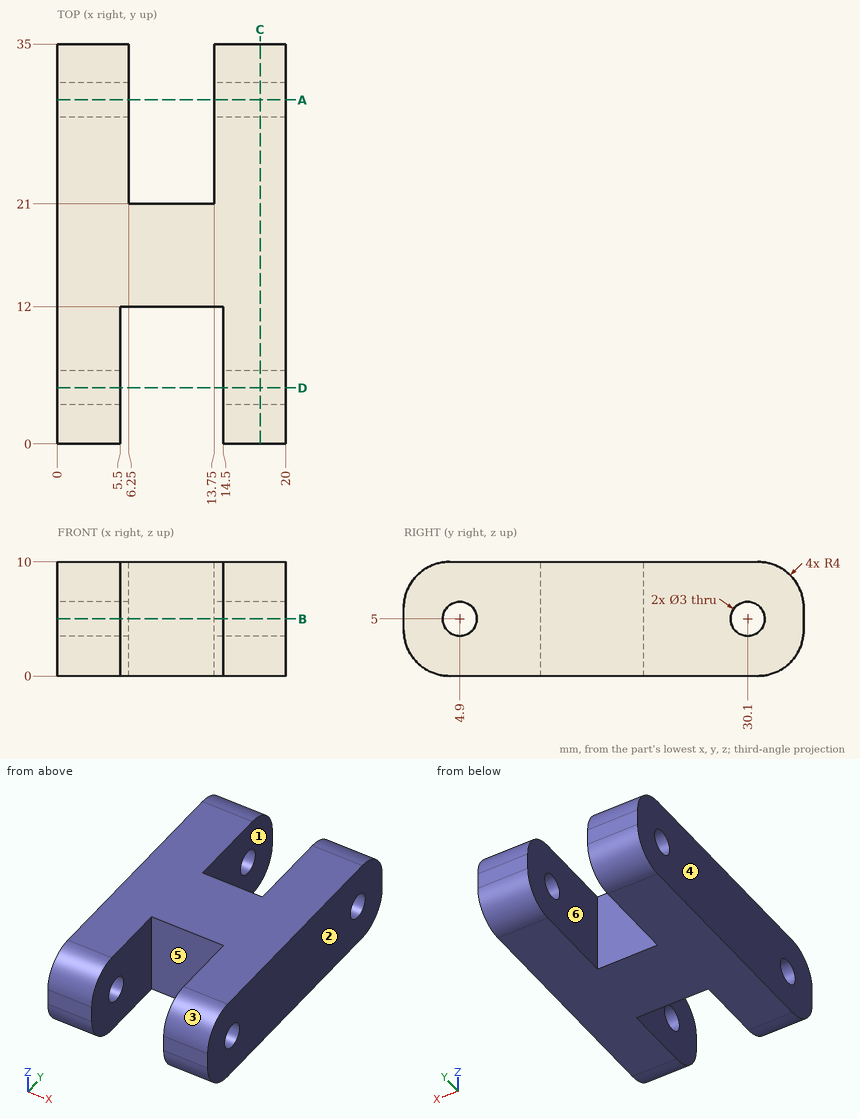
Could you check a few things on this drawing? It's one solid part, dimensions in mm from its lowest x, y, z. A direction names the side the tool comes from. Give positions to 0.01 mm unless a question says otherwise; leave off trailing zeros. Loops run counter-clockwise (first coordinate to the right, second up) from the corner with the lowest first, then second, coordinate; pieces in that order, holes last. Notation, with made-up numbers: M -38.75,12.25 L 1.25,12.25 A14 cw 1.25,19.25 Z; hole C 22.25,8.25 d5. An arc over 180 degrees is marked long. One line per question, with ' | ' between items. Start each with the question number.
Q1. If I drill on line 1 (Y direction, x = 4.15, z = 5); line 2 (Z direction, x = 3.5, y = 30.1); line 3 (X direction, y = 4.5, z = 9.75), over which ranges is the centre line in solid material (lowest first)? Write a range as from..to.
Q2. For the marked faces 4, 5 and 6, which set-ups out of +Z, -Z, +X, -X, +Y, -Y let a thin tool reach every point of the face, with its end or its side?
Q3. If we section it at C-C (x = 17.75): Please give me the cut outline in (y, z).
Q4. If we section it at B-B (z = 5): Please give me the cut outline in (x, y).
Q5. If we section it at A-A (y = 30.1): Please give me the cut outline in (x, z), plus the area to 3 significant figures.
Q6. If we mould it in two halves opening along X, with no side actions, what happens to the marked faces 1, 2 and 3? For each: +X half, -X half, draft (parallel to the pull), parting line (faces both ways), or undercut.
Q7. For pin 1 Ø1.5 at (x, z) = (6.5, 7) entering from -Y; pin 2 Ø1.5 at (x, z) = (10, 2) entering from +Y, each with a flat end and sliding along its axis, tell me the tip position at first contact or that it passes through.
Q8. If we section it at D-D (y = 4.9): Please give me the cut outline in (x, z), plus the area to 3 significant figures.
Computed:
1) line 1: y = 0..3.4, 6.4..28.6, 31.6..35 | line 2: z = 0..3.5, 6.5..10 | line 3: x = 0..5.5, 14.5..20
2) face 4: +Z, -Z, -X, +Y, -Y | face 5: +Z, -Z, -Y | face 6: +Z, -Z, +Y
3) outline: M 0,4 A4 ccw 4,0 L 31,0 A4 ccw 35,4 L 35,6 A4 ccw 31,10 L 4,10 A4 ccw 0,6 Z; hole C 4.9,5 d3; hole C 30.1,5 d3
4) outline: M 0,0 L 5.5,0 L 5.5,3.4 L 0,3.4 Z; M 0,6.4 L 5.5,6.4 L 5.5,12 L 14.5,12 L 14.5,6.4 L 20,6.4 L 20,28.6 L 13.75,28.6 L 13.75,21 L 6.25,21 L 6.25,28.6 L 0,28.6 Z; M 0,31.6 L 6.25,31.6 L 6.25,35 L 0,35 Z; M 13.75,31.6 L 20,31.6 L 20,35 L 13.75,35 Z; M 14.5,0 L 20,0 L 20,3.4 L 14.5,3.4 Z
5) outline: M 0,0 L 6.25,0 L 6.25,3.5 L 0,3.5 Z; M 0,6.5 L 6.25,6.5 L 6.25,10 L 0,10 Z; M 13.75,0 L 20,0 L 20,3.5 L 13.75,3.5 Z; M 13.75,6.5 L 20,6.5 L 20,10 L 13.75,10 Z | area: 87.5 mm²
6) face 1: undercut | face 2: +X half | face 3: draft
7) pin 1: stops at y = 12 | pin 2: stops at y = 21
8) outline: M 0,0 L 5.5,0 L 5.5,3.5 L 0,3.5 Z; M 0,6.5 L 5.5,6.5 L 5.5,10 L 0,10 Z; M 14.5,0 L 20,0 L 20,3.5 L 14.5,3.5 Z; M 14.5,6.5 L 20,6.5 L 20,10 L 14.5,10 Z | area: 77.0 mm²
